Can you work these out from the model? Positions are in its coordinate system, mm. A direction names the side the tool comes from. Give positions to 0.01 mm unless a question says otherwise; leave off trailing zeros. Loops run counter-clockwise (first coordinate to the right, second up) from the corner with the lowest first, then second, coordinate; pieces in that order, holes last. Notation, with made-up numbers: M -1,-15.75 L 54,-15.75 A28 ccw 54,7.25 Z; hole C 80,76 d5. An arc over 180 degrees is marked long. Answer as a JSON object with one key per item and string values.
```python
from build123d import *

# Parameters (mm, degrees)
BOSS_EXTRUDE1_DEPTH = 12.7
SKETCH2_W           = 8.89
SKETCH2_H           = 1.5875
BOSS_EXTRUDE2_DEPTH = 12.7
SKETCH3_R           = 1.5875
CUT_EXTRUDE1_DEPTH  = 17.78


with BuildPart() as part:
    # Sketch1 → Boss-Extrude1 (new body)
    # profile 1 of 3: a face of its own
    with BuildSketch(Plane.XY):
        with BuildLine():
            ThreePointArc((0, -1.5875), (-1.5875, -1.162130657), (-2.749630657, 0))
            Line((-2.749630657, 0), (-12.7, 0))
            Line((-12.7, 0), (-12.7, -1.5875))
            Line((-12.7, -1.5875), (0, -1.5875))
        make_face()
    # profile 2 of 3: a face of its own
    with BuildSketch(Plane.XY):
        with BuildLine():
            Line((0, -1.5875), (0, 0))
            Line((0, 0), (-2.749630657, 0))
            ThreePointArc((-2.749630657, 0), (-1.5875, -1.162130657), (0, -1.5875))
        make_face()
    # profile 3 of 3: a face of its own
    with BuildSketch(Plane.XY):
        with BuildLine():
            Line((-2.749630657, 0), (0, 0))
            Line((0, 0), (0, -1.5875))
            ThreePointArc((0, -1.5875), (2.24506403, -0.65756403), (3.175, 1.5875))
            ThreePointArc((3.175, 1.5875), (-0.821750468, 4.654314498), (-2.749630657, 0))
        make_face()
        with BuildLine():
            ThreePointArc((1.5875, 1.5875), (1.122532015, 0.464967985), (0, 0))
            ThreePointArc((0, 0), (-1.122532015, 2.710032015), (1.5875, 1.5875))
        make_face(mode=Mode.SUBTRACT)
    extrude(amount=BOSS_EXTRUDE1_DEPTH)

    # Sketch2 → Boss-Extrude2 (add)
    with BuildSketch(Plane(origin=(0, 0, 0), x_dir=(-1, 0, 0), z_dir=(0, 0, -1))):
        with Locations((8.255, -0.79375)):
            Rectangle(SKETCH2_W, SKETCH2_H)
    extrude(amount=BOSS_EXTRUDE2_DEPTH)

    # Sketch3 → Cut-Extrude1 (cut)
    with BuildSketch(Plane(origin=(0, 0, 0), x_dir=(1, 0, 0), z_dir=(0, 1, 0))):
        with Locations(Location((-7.874, 7.874, 0), (0, 0, 180))):
            Circle(SKETCH3_R)
        with Locations(Location((-7.874, -7.874, 0), (0, 0, 180))):
            Circle(SKETCH3_R)
    extrude(amount=-CUT_EXTRUDE1_DEPTH, mode=Mode.SUBTRACT)


solid = part.part
```
1) Suppose I cut it at C-C, the plane z = -8.5. Write out the boundary of the cut face in (x, y), and give its area (3 significant figures).
Answer list:
{"outline": "M -12.7,-1.59 L -9.33,-1.59 L -9.33,0 L -12.7,0 Z; M -6.42,-1.59 L -3.81,-1.59 L -3.81,0 L -6.42,0 Z", "area": "9.48 mm^2"}
2) Please list where these lines run through material, in increasing order: line 1 along Z through (x, y) = (-7.5, -0.5); line 2 along X through (y, z) = (1.75, 8.5); line 3 along X through (y, z) = (2.75, 1). Write a range as from..to.
Answer list:
{"line 1": "-12.7..-9.42, -6.33..6.33, 9.42..12.7", "line 2": "-3.17..-1.58, 1.58..3.17", "line 3": "-2.95..-1.08, 1.08..2.95"}
3) If we mould it in two halves opening along X, with no side actions, what happens to faces 1 (the cylindrical face through (-8.607, -0.783, 6.466)), 2 (the flat face through (-12.7, -1, 0)), 3 (the flat face through (-3.81, -1, -6)), 4 (the flat face through (-3.1, -0.5, 12.7))? For each: +X half, -X half, draft (parallel to the pull), parting line (faces both ways), or undercut.
Answer list:
{"face 1": "undercut", "face 2": "-X half", "face 3": "+X half", "face 4": "draft"}
4) For faces 5 (the flat face through (-1, 0, 0)), 6 (the flat face through (-6, -1.588, 0)), which set-ups out of +Z, -Z, +X, -X, +Y, -Y let a thin tool reach every point of the face, with its end or its side?
Answer list:
{"face 5": "-Z, +X, +Y, -Y", "face 6": "+Z, -Z, +X, -X, -Y"}
5) Will these pins go through, and if not, where does the flat tip stop? pin 1 Ø3 at (y, z) = (1, -0.5) entering from +X (3 decimals); pin 2 Ø6 at (x, z) = (-8, 6) entering from +Y; pin 3 Ø1.5 at (y, z) = (1, 8.5) entering from -X (3 decimals); pin 4 Ø0.8 at (y, z) = (-0.5, -5.5) entering from +X.
Answer list:
{"pin 1": "x = 3.175", "pin 2": "y = 0", "pin 3": "x = -3.175", "pin 4": "x = -3.81"}
6) Suppose I cut it at D-D, the plane x = -8.5. Write out the boundary of the cut face in (y, z).
Answer list:
{"outline": "M -1.59,-12.7 L 0,-12.7 L 0,-9.33 L -1.59,-9.33 Z; M -1.59,-6.42 L 0,-6.42 L 0,6.42 L -1.59,6.42 Z; M -1.59,9.33 L 0,9.33 L 0,12.7 L -1.59,12.7 Z"}
7) Suppose I cut it at B-B, the plane x = 0.5. Write out the boundary of the cut face in (y, z), and give its area (3 significant figures).
Answer list:
{"outline": "M -1.55,0 L 0.08,0 L 0.08,12.7 L -1.55,12.7 Z; M 3.09,0 L 4.72,0 L 4.72,12.7 L 3.09,12.7 Z", "area": "41.4 mm^2"}
